Part model, mm, in its own coordinate system. A direction names the side the tool comes from. Give positions to 0.01 mm unless a question says otherwise; leave off trailing zeros. Order: outer loops, then holes, each group sorted by start corner. A loop starts at its lowest first (then second) coordinate and runs counter-clockwise, first axis right, second up. Notation, with made-up numbers: (73.25, 45) -> (94.25, 45) arc R25 cw to (94.25, 76) -> close; hole circle Ø5 at (26, -9.5). An arc over 180 degrees is marked (long way). Write item = value, one per line. Start each with the question number.
(1) Probe line 1 along Y through (x, z) = (-98, 8.5) (1 decimal); line 2 along Y through (x, z) = (-107.5, 2.5) (1 decimal); line 3 along Z through (x, y) = (-227, -11). List the from-to ranges inside material, lowest first. Write a range as from..to.
(2) Saw through at C-C, the plane y = -12. List the corners of the cut face in (x, z) (3 decimals).
(3) Saw through at B-B, the plane y = -46. List the corners of the cut face in (x, z) (3 decimals).
(4) Flat gauge pins, fed straight in: pin 1 (6 mm diameter, centred on x = 59.51, y = 44.15, fed in from -Z); pin 2 (1.4 mm diameter, centred on y = 3.5, z = 13.5, fed in from +X) (3 decimals); pin 3 (3 mm diameter, centred on x = 188.6, z = 5.88, fed in from +Y); pin 4 (10 mm diameter, centred on x = -196, y = 8.5, fed in from -Z). Where does each tip first touch, or does it go through?
(5) Which spindle directions (+Z, -Z, +X, -X, +Y, -Y) get a long thin tool onto all of the face, cutting with end or side? Do faces 1 (the flat face through (-4, 46, 2.756)), 2 (the flat face through (4, -51.879, 6)), 3 (the flat face through (320.675, 35, 7)). Say none if no direction does.
(6) Two-plate mould, pull along X, no slides. Class faces 4 (the cylindrical face through (257.55, 3.42, 13.12)), 5 (the flat face through (-320.675, 35, 7)), 6 (the cylindrical face through (-257.14, 1.08, 13.12)), 7 (the flat face through (-4, -53.975, 7)): pulls with the +X half, pulls with the -X half, needs draft (parallel to the pull), parting line crosses it, or undercut.
(7) Saw through at A-A, the plane x = 116.5. List the corners of the cut face in (y, z) (1 decimal).
from build123d import *

# Parameters (mm, degrees)
SKETCH1_W           = 641.35
SKETCH1_H           = 107.95
BOSS_EXTRUDE1_DEPTH = 14.5161
SKETCH2_W           = 641.35
SKETCH2_H           = 17.78
CUT_EXTRUDE1_DEPTH  = 11.7602
SKETCH3_W           = 641.35
SKETCH3_H           = 85.5345
CUT_EXTRUDE3_DEPTH  = 11.7602
FILLET1_R           = 2.032
CUT_EXTRUDE4_DEPTH  = 326.398307546
SKETCH5_R           = 3.429
CUT_EXTRUDE5_DEPTH  = 11.7602
SKETCH6_R           = 5.461
CUT_EXTRUDE6_DEPTH  = 11.7602
SKETCH7_R           = 2.54
CUT_EXTRUDE7_DEPTH  = 2.54


with BuildPart() as part:
    # Sketch1 → Boss-Extrude1 (new body)
    with BuildSketch(Plane.XY):
        Rectangle(SKETCH1_W, SKETCH1_H)
    extrude(amount=BOSS_EXTRUDE1_DEPTH)

    # Sketch2 → Cut-Extrude1 (cut)
    with BuildSketch(Plane.XY.offset(14.5161)):
        with Locations((0, 45.085)):
            Rectangle(SKETCH2_W, SKETCH2_H)
    extrude(amount=-CUT_EXTRUDE1_DEPTH, mode=Mode.SUBTRACT)

    # Sketch3 → Cut-Extrude3 (cut)
    with BuildSketch(Plane(origin=(0, 0, 0), x_dir=(-1, 0, 0), z_dir=(0, 0, -1))):
        with Locations((0, -9.11225)):
            Rectangle(SKETCH3_W, SKETCH3_H)
    extrude(amount=-CUT_EXTRUDE3_DEPTH, mode=Mode.SUBTRACT)

    # Fillet1
    fillet1_edges = [part.edges().sort_by_distance(p)[0] for p in [
        (0, 36.195, 2.7559),
        (0, 33.655, 0),
    ]]
    fillet(fillet1_edges, radius=FILLET1_R)

    # Sketch4 → Cut-Extrude4 (cut, through all)
    with BuildSketch(Plane(origin=(0, 0, 11.7602), x_dir=(-1, 0, 0), z_dir=(0, 0, -1))):
        with BuildLine():
            Line((-294.005, 19.685), (-320.675, 19.685))
            Line((-320.675, 19.685), (-320.675, -29.845))
            Line((-320.675, -29.845), (-294.005, -29.845))
            ThreePointArc((-294.005, -29.845), (-289.514871939, -27.985128061), (-287.655, -23.495))
            Line((-287.655, -23.495), (-287.655, 13.335))
            ThreePointArc((-287.655, 13.335), (-289.514871939, 17.825128061), (-294.005, 19.685))
        make_face()
        with BuildLine():
            Line((294.005, -29.845), (320.675, -29.845))
            Line((320.675, -29.845), (320.675, 19.685))
            Line((320.675, 19.685), (294.005, 19.685))
            ThreePointArc((294.005, 19.685), (289.514871939, 17.825128061), (287.655, 13.335))
            Line((287.655, 13.335), (287.655, -23.495))
            ThreePointArc((287.655, -23.495), (289.514871939, -27.985128061), (294.005, -29.845))
        make_face()
    extrude(amount=-CUT_EXTRUDE4_DEPTH, mode=Mode.SUBTRACT)

    # Sketch5 → Cut-Extrude5 (cut)
    with BuildSketch(Plane(origin=(0, 0, 0), x_dir=(-1, 0, 0), z_dir=(0, 0, -1))):
        with Locations((-279.222061941, 44.148206771)):
            Circle(SKETCH5_R)
        with Locations((-235.280061941, 44.148206771)):
            Circle(SKETCH5_R)
        with Locations((-191.338061941, 44.148206771)):
            Circle(SKETCH5_R)
        with Locations((-147.396061941, 44.148206771)):
            Circle(SKETCH5_R)
        with Locations((-103.454061941, 44.148206771)):
            Circle(SKETCH5_R)
        with Locations((-59.512061941, 44.148206771)):
            Circle(SKETCH5_R)
        with Locations((-15.570061941, 44.148206771)):
            Circle(SKETCH5_R)
        with Locations((28.371938059, 44.148206771)):
            Circle(SKETCH5_R)
        with Locations((72.313938059, 44.148206771)):
            Circle(SKETCH5_R)
        with Locations((116.255938059, 44.148206771)):
            Circle(SKETCH5_R)
        with Locations((160.197938059, 44.148206771)):
            Circle(SKETCH5_R)
        with Locations((204.139938059, 44.148206771)):
            Circle(SKETCH5_R)
        with Locations((248.081938059, 44.148206771)):
            Circle(SKETCH5_R)
        with Locations((287.655, 44.148206771)):
            Circle(SKETCH5_R)
    extrude(amount=-CUT_EXTRUDE5_DEPTH, mode=Mode.SUBTRACT)

    # Sketch6 → Cut-Extrude6 (cut)
    with BuildSketch(Plane(origin=(0, 0, 11.7602), x_dir=(-1, 0, 0), z_dir=(0, 0, -1))):
        with Locations((-252.095, 3.175)):
            Circle(SKETCH6_R)
        with Locations((252.095, 3.175)):
            Circle(SKETCH6_R)
    extrude(amount=-CUT_EXTRUDE6_DEPTH, mode=Mode.SUBTRACT)

    # Sketch7 → Cut-Extrude7 (cut)
    with BuildSketch(Plane(origin=(0, -51.8795, 0), x_dir=(1, 0, 0), z_dir=(0, 1, 0))):
        with Locations(Location((-206.375, -5.8801, 0), (0, 0, 180))):
            Circle(SKETCH7_R)
        with Locations(Location((-197.485, -5.8801, 0), (0, 0, 180))):
            Circle(SKETCH7_R)
        with Locations(Location((-188.595, -5.8801, 0), (0, 0, 180))):
            Circle(SKETCH7_R)
        with Locations(Location((197.485, -5.8801, 0), (0, 0, 270))):
            Circle(SKETCH7_R)
        with Locations(Location((188.595, -5.8801, 0), (0, 0, 270))):
            Circle(SKETCH7_R)
        with Locations(Location((206.375, -5.8801, 0), (0, 0, 270))):
            Circle(SKETCH7_R)
    extrude(amount=-CUT_EXTRUDE7_DEPTH, mode=Mode.SUBTRACT)


solid = part.part
Results list:
q1.line_1 = -54..-51.9, 33.7..36.2
q1.line_2 = -54..-51.9, 33.7..54
q1.line_3 = 11.76..14.52
q2.outline = (-287.655, 11.76) -> (287.655, 11.76) -> (287.655, 14.516) -> (-287.655, 14.516) -> close
q3.outline = (-320.675, 11.76) -> (320.675, 11.76) -> (320.675, 14.516) -> (-320.675, 14.516) -> close
q4.pin_1 = through
q4.pin_2 = 287.655
q4.pin_3 = 36.24
q4.pin_4 = 11.76
q5.face_1 = +Z, +X, -X, +Y
q5.face_2 = -Z, +X, -X
q5.face_3 = +Z, -Z, +X, +Y, -Y
q6.face_4 = undercut
q6.face_5 = pulls with the -X half
q6.face_6 = undercut
q6.face_7 = needs draft
q7.outline = (-54, 0) -> (-51.9, 0) -> (-51.9, 11.8) -> (33.7, 11.8) -> (33.7, 2) arc R2 ccw to (35.7, 0) -> (54, 0) -> (54, 2.8) -> (38.2, 2.8) arc R2 cw to (36.2, 4.8) -> (36.2, 14.5) -> (-54, 14.5) -> close
